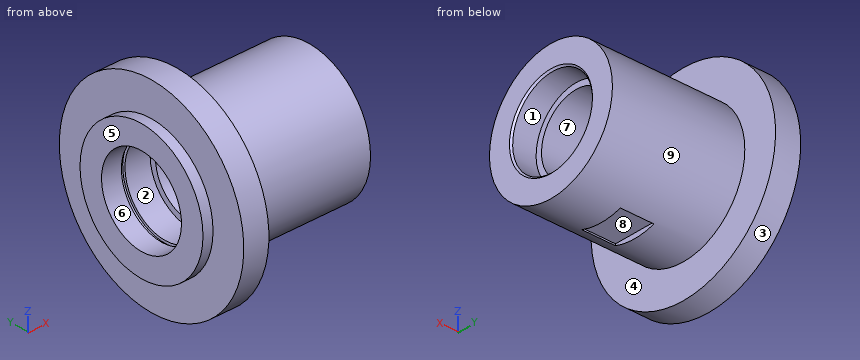
```python
from build123d import *

# Parameters (mm, degrees)
SKETCH2_W                                           = 20
SKETCH2_H                                           = 24.98
CUT_EXTRUDE1_DEPTH                                  = 3
CBORE_FOR_M5_HEX_SOCKET_HEAD_CAP_SCREW1_D           = 45
CBORE_FOR_M5_HEX_SOCKET_HEAD_CAP_SCREW1_CBORE_D     = 52
CBORE_FOR_M5_HEX_SOCKET_HEAD_CAP_SCREW1_CBORE_DEPTH = 15
CHAMFER1_SIZE                                       = 1
CUT_EXTRUDE2_START                                  = -29
SKETCH15_R                                          = 26
CUT_EXTRUDE2_DEPTH                                  = 29
SKETCH16_W                                          = 2.15
SKETCH16_H                                          = 27.5


with BuildPart() as part:
    # Sketch1 → Revolve1 (revolve)
    with BuildSketch(Plane.XY, mode=Mode.PRIVATE) as revolve1_sk:
        Polygon((0, 0), (0, 40), (6, 40), (6, 60), (21, 60), (21, 40), (100, 40), (100, 0), align=None)
    revolve(revolve1_sk.sketch.rotate(Axis((0, 0, 0), (1, 0, 0)), 90), axis=Axis((0, 0, 0), (1, 0, 0)))

    # Sketch2 → Cut-Extrude1 (cut)
    with BuildSketch(Plane(origin=(0, 0, -40), x_dir=(-1, 0, 0), z_dir=(0, 0, -1))):
        with Locations((-60, 0)):
            Rectangle(SKETCH2_W, SKETCH2_H)
    extrude(amount=-CUT_EXTRUDE1_DEPTH, mode=Mode.SUBTRACT)

    # CBORE for M5 Hex Socket Head Cap Screw1 (through all)
    with Locations(Plane(origin=(100, 0, 0), x_dir=(0, 0, -1), z_dir=(1, 0, 0))):
        with Locations((0, 0)):
            CounterBoreHole(CBORE_FOR_M5_HEX_SOCKET_HEAD_CAP_SCREW1_D / 2, CBORE_FOR_M5_HEX_SOCKET_HEAD_CAP_SCREW1_CBORE_D / 2, CBORE_FOR_M5_HEX_SOCKET_HEAD_CAP_SCREW1_CBORE_DEPTH)

    # Chamfer1
    chamfer1_edges = [part.edges().sort_by_distance(p)[0] for p in [
        (100, 0, 26),
    ]]
    chamfer(chamfer1_edges, length=CHAMFER1_SIZE)

    # Sketch15 → Cut-Extrude2 (cut)
    with BuildSketch(Plane.ZY.offset(CUT_EXTRUDE2_START)):
        with Locations(Location((0, 0, 0), (0, 0, 180))):
            Circle(SKETCH15_R)
    extrude(amount=CUT_EXTRUDE2_DEPTH, mode=Mode.SUBTRACT)

    # Sketch16 → Cut-Revolve1 (revolve, cut)
    with BuildSketch(Plane.XY, mode=Mode.PRIVATE) as cut_revolve1_sk:
        with Locations((12.925, 13.75)):
            Rectangle(SKETCH16_W, SKETCH16_H)
    revolve(cut_revolve1_sk.sketch.rotate(Axis((0, 0, 0), (1, 0, 0)), 90), axis=Axis((0, 0, 0), (1, 0, 0)), mode=Mode.SUBTRACT)


solid = part.part
```
The listing builds one solid part. Answer for the finished solid, in the listing's coordinates (mm). Face numbers are marked on the shaded views. A direction names the side the tool comes from. Coordinates: 2 decimals unless noted, no trailing zeros. Order: outer loops, then holes, each group sorted by start corner. A loop starts at its lowest first (then second) coordinate and runs counter-clockwise, first axis right, second up. Notation, with made-up numbers: M 45.5,23.25 L 69.5,23.25 A33 cw 69.5,57.25 Z; hole C 63.5,3 d3. An arc over 180 degrees is marked long. Answer as a JSON object with one key per item and string values. Group by question number.
1. A tool of negligible diameter and unlimited length cuts with its end or side. For the marked faces 5, 6, 7, 8 and 9, from which of +Z, -Z, +X, -X, +Y, -Y can it reach the whole face along a straight path? Write none if from no direction.
2. Section B-B on x = 92 is taken. Write down the section's boundary in (y, z), then the cut area to 3 significant figures.
3. Flat-ended cylindrical pins translate along their axes: P1, Ø8, axis at x = 88.5, z = -34, coming from the -Y side; P2, Ø12, axis at x = 21.5, z = 18, coming from the +Y side; P3, Ø0.8, axis at x = 56, z = -37.5, coming from the -Y side. Find the tip coordinate at first contact, or state that the pin passes through.
4. Section C-C on y = -32 is taken. Write down the section's boundary in (x, z).
5. Straight lines are drawn through the part: line 1 (Y direction, x = 54.5, z = 0); line 2 (X direction, y = 7, z = 42); line 3 (Z direction, x = 5, y = -17.5). For each, find the intervals that lie inside material, in ascending order.
6. Determine the mould class of the marked faces 1, 2, 3 and 4 for opening direction Z: released by +Z, released by -Z, zero draft, split by the parting line, or undercut.
Values follow:
{
 "1": {"face 5": "+Z, -Z, -X, +Y, -Y", "face 6": "-X", "face 7": "+X, -X", "face 8": "-Z", "face 9": "+X"},
 "2": {"outline": "C 0,0 d80; hole C 0,0 d52", "area": "2,900 mm2"},
 "3": {"P1": "y = -26.46", "P2": "y = 58.78", "P3": "y = -14.95"},
 "4": {"outline": "M 0,-24 L 6,-24 L 6,-50.75 L 21,-50.75 L 21,-24 L 100,-24 L 100,24 L 21,24 L 21,50.75 L 6,50.75 L 6,24 L 0,24 Z"},
 "5": {"line 1": "-40 to -22.5, 22.5 to 40", "line 2": "6 to 21", "line 3": "-35.97 to -19.23, 19.23 to 35.97"},
 "6": {"face 1": "undercut", "face 2": "undercut", "face 3": "split by the parting line", "face 4": "zero draft"}
}
